Geometry: see drawing. Coordinates: mm, zero at the bounding-box minimum. Give positions to 0.01 mm unless a question says otherwise; leave off trailing zeros. Write each loop counter-clockwise with the first axis right and the second up, starting at its lowest first coordinate (ties: lowest second). Pieces come first, ordered by that corner, then holes.
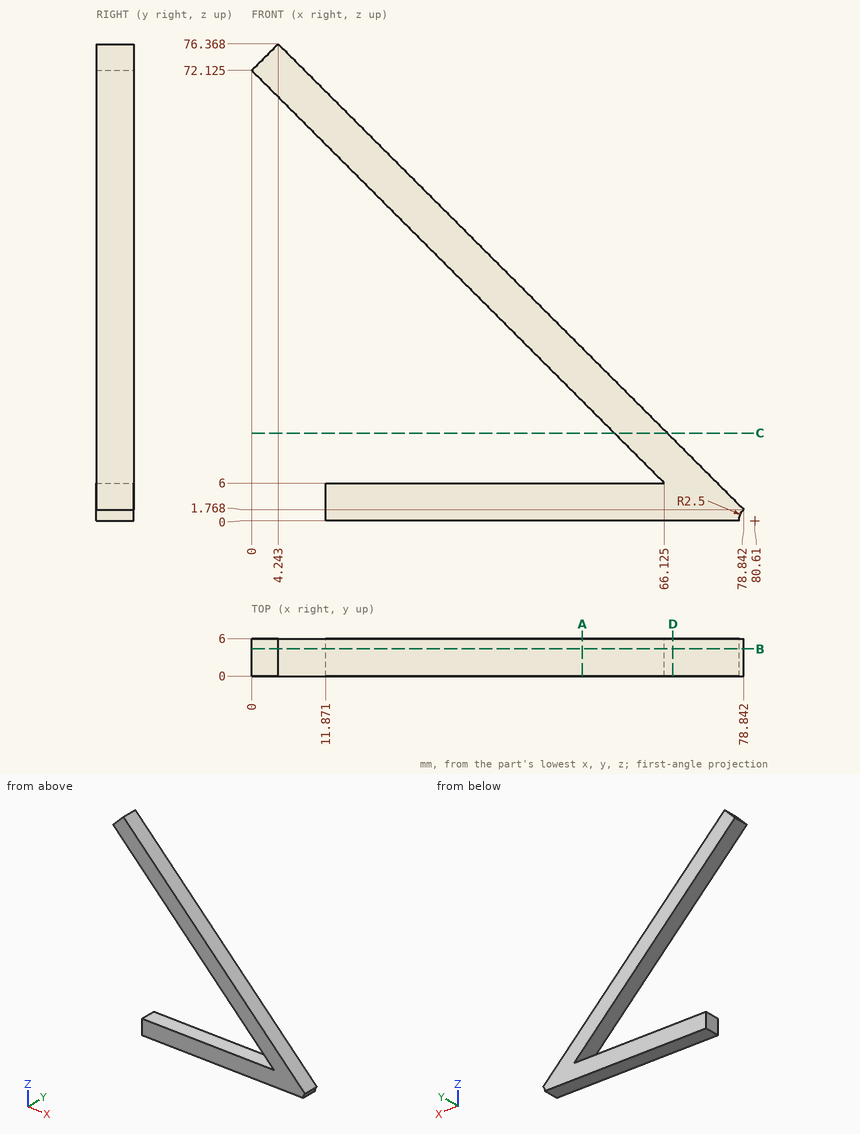
1. Line query: probe 1 along Z at (x, y) = (49, 4.95) (1 decimal); probe 2 along Z at (x, y) = (35, 5.65) (1 decimal); probe 3 along X at (y, z) = (2.2, 65) (1 decimal). Output: solid intervals per line, ascending.
2. Section query D-D (x = 67.5). Return loops of the section in (y, z).
3. Section query C-C (z = 14). Return loops of the section in (x, y) (1 decimal).
4. Section query A-A (x = 53). Return loops of the section in (y, z) (1 decimal).
5. Section query B-B (y = 4.35). Return loops of the section in (x, z) (1 decimal).
6. Pin query (flat end, axial travel): P1, Ø4, axis at x = 35.5, z = 9, coming from the +Y side; P2, Ø3, axis at y = 3, z = 4.5, coming from the -X side; P3, Ø2, axis at y = 3.5, z = 40, coming from the +X side; P4, Ø3, axis at x = 25, y = 1.5, coming from the +Z side. Return the tip coordinate at first contact, or that it passes through.
The answers:
1. probe 1: z = 0 to 6, 23.1 to 31.6
1. probe 2: z = 0 to 6, 37.1 to 45.6
1. probe 3: x = 7.1 to 15.6
2. outline: (0, 0) - (6, 0) - (6, 13.11) - (0, 13.11) - close
3. outline: (58.1, 0) - (66.6, 0) - (66.6, 6) - (58.1, 6) - close
4. outline: (0, 0) - (6, 0) - (6, 6) - (0, 6) - close; (0, 19.1) - (6, 19.1) - (6, 27.6) - (0, 27.6) - close
5. outline: (0, 72.1) - (66.1, 6) - (11.9, 6) - (11.9, 0) - (78.1, 0) arc R2.5 cw to (78.8, 1.8) - (4.2, 76.4) - close
6. P1: passes through
6. P2: stops at x = 11.87
6. P3: stops at x = 41.61
6. P4: stops at z = 57.11
